The figure shows three views and two pictorial views of one solid part (mm, origin at its lowest corner). Answer the questions. Coordinates: 2 decimals unless noted, no trailing zeros. Loops run counter-clockwise (first coordinate to the right, second up) from the corner with the lowest first, then second, coordinate; pieces in that order, holes last. Notation, with made-up numbers: (-12.5, 24) -> (11.5, 24) arc R33 ccw to (11.5, 53) -> close; hole circle Ø9 at (26, 0). An arc over 180 degrees is marked (long way). Answer as a JSON object with one key per item and string values. Group by question number.
1) Section B-B, the plane x = 24.5 is taken. Give the vertices of the cut face in (y, z), plus the area to 3 significant figures.
2) Determine the mould class of the marked faces 1 and 2 for opening direction Y: released by +Y, released by -Y, zero draft, split by the parting line, or undercut.
3) Flat-ended cylindrical pins translate along their axes: P1, Ø2, axis at x = 20.88, y = 25, coming from the -Z side; P2, Ø4, axis at x = 7, z = 7.5, coming from the +Y side; P3, Ø4, axis at y = 8, z = 8, coming from the -X side; P4, Ø4, axis at x = 35.5, z = 12, coming from the +Y side. Find the tip coordinate at first contact, or state that the pin passes through.
4) Section D-D, the plane x = 5 is taken. Give the vertices of the cut face in (y, z), plus the area to 3 significant figures.
5) Section C-C, the plane y = 20 is taken. Give the vertices of the cut face in (x, z).
6) Section A-A, the plane z = 6.75 is taken. Give the vertices of the cut face in (x, y).
7) Consider probe 1 along X at (y, z) = (25, 17.4); probe 2 along Y at (x, z) = (41.5, 12.25) (1 decimal); probe 3 along Y at (x, z) = (2, 8.5). Determine where each line is inside the solid, lowest interval first. Write a range as [from, to].
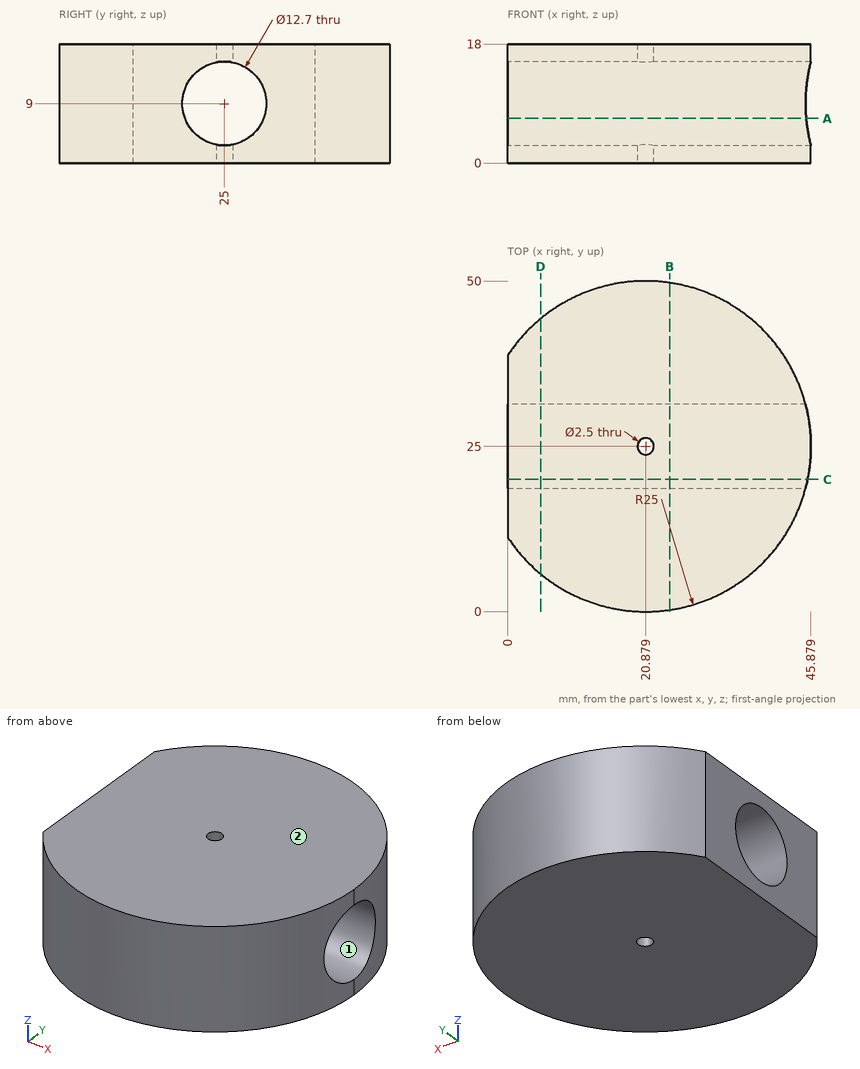
Determined:
{
 "1": {"outline": "(0.26, 0) -> (49.74, 0) -> (49.74, 18) -> (0.26, 18) -> close; hole circle Ø12.7 at (25, 9)", "area": "764 mm²"},
 "2": {"face 1": "undercut", "face 2": "zero draft"},
 "3": {"P1": "through", "P2": "y = 47", "P3": "x = 0.88", "P4": "y = 46.58"},
 "4": {"outline": "(5.69, 0) -> (44.31, 0) -> (44.31, 18) -> (5.69, 18) -> close; hole circle Ø12.7 at (25, 9)", "area": "568 mm²"},
 "5": {"outline": "(0, 0) -> (45.37, 0) -> (45.37, 5.09) -> (0, 5.09) -> close; (0, 12.91) -> (45.37, 12.91) -> (45.37, 18) -> (0, 18) -> close"},
 "6": {"outline": "(0, 11.25) arc R25 ccw to (45.16, 19.06) -> (0, 19.06) -> close; (0, 30.94) -> (45.16, 30.94) arc R25 ccw to (0, 38.75) -> close"},
 "7": {"probe 1": "[0, 19.63], [22.13, 45.88]", "probe 2": "[10.9, 19.5], [30.5, 39.1]", "probe 3": "[8.61, 18.67], [31.33, 41.39]"}
}
